Verification items for this drawing (mm, ordinates from the low corner). Give positions to 0.01 mm unless a question says otherwise; leave off trailing zeros. Loops run counter-clockwise (first coordinate to the right, second up) from the corner with the lowest first, then second, coordinate; pieces in that order, holes last. Notation, with made-up numbers: (77.25, -35.75) - (123.25, -35.75) arc R18 ccw to (123.25, -6.75) - close; hole circle Ø4 at (26, 61.5). An arc over 180 degrees is marked (long way). One line per question, with ' | ' between items. Start each with the question number.
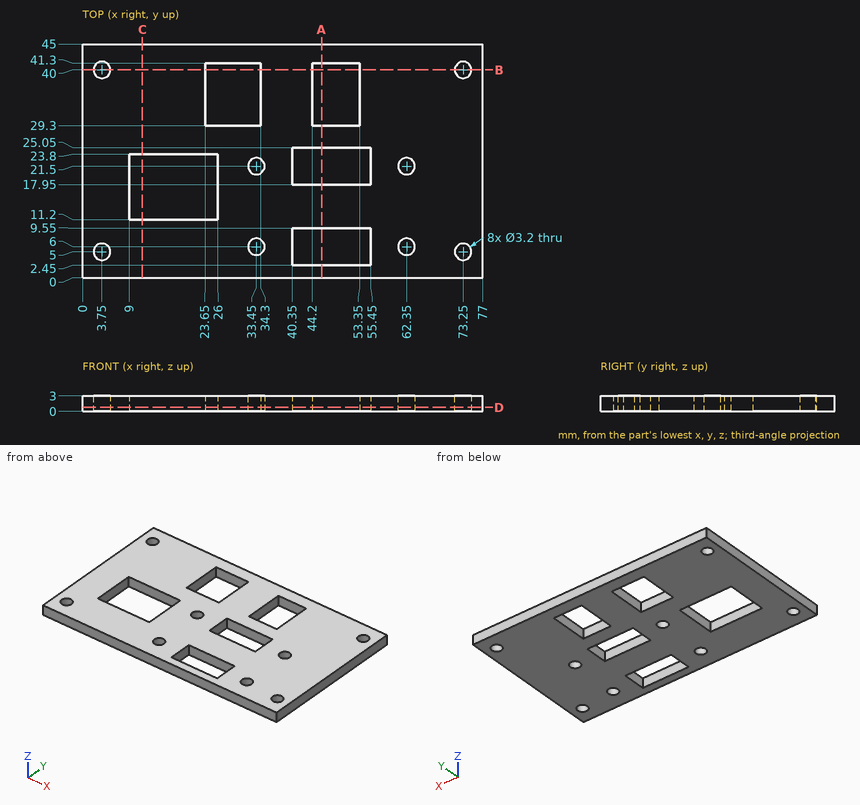
(1) Section check A-A, the plane x = 46. Record the boundary of the cut face in (y, z), and give its area (3 significant figures).
(2) Section check C-C, the plane x = 11.5. Record the boundary of the cut face in (y, z), and give its area (3 significant figures).
(3) Section check B-B, the plane y = 40. Record the boundary of the cut face in (x, z), and give its area (3 significant figures).
(4) Section check D-D, the plane z = 0.8. Count the separate pieces of the cut face and the enclosed holes in it, and give its area (3 significant figures).
(5) Material ranges on line 1 (Y direction, x = 62.35, z = 1.45); line 2 (X direction, y = 36.5, z = 2.1); line 3 (Y direction, x = 3.75, z = 0.95), recorded low to high.
Numbers:
1) outline: (0, 0) - (2.45, 0) - (2.45, 3) - (0, 3) - close; (9.55, 0) - (17.95, 0) - (17.95, 3) - (9.55, 3) - close; (25.05, 0) - (29.3, 0) - (29.3, 3) - (25.05, 3) - close; (41.3, 0) - (45, 0) - (45, 3) - (41.3, 3) - close | area: 56.4 mm^2
2) outline: (0, 0) - (11.2, 0) - (11.2, 3) - (0, 3) - close; (23.8, 0) - (45, 0) - (45, 3) - (23.8, 3) - close | area: 97.2 mm^2
3) outline: (0, 0) - (2.15, 0) - (2.15, 3) - (0, 3) - close; (5.35, 0) - (23.65, 0) - (23.65, 3) - (5.35, 3) - close; (34.3, 0) - (44.2, 0) - (44.2, 3) - (34.3, 3) - close; (53.35, 0) - (71.65, 0) - (71.65, 3) - (53.35, 3) - close; (74.85, 0) - (77, 0) - (77, 3) - (74.85, 3) - close | area: 152 mm^2
4) separate pieces: 1 | enclosed holes: 13 | area: 2,730 mm^2
5) line 1: 0 to 4.4, 7.6 to 19.9, 23.1 to 45 | line 2: 0 to 23.65, 34.3 to 44.2, 53.35 to 77 | line 3: 0 to 3.4, 6.6 to 38.4, 41.6 to 45
